from build123d import *

# Parameters (mm, degrees)
F0_W     = 203.2
F0_H     = 304.8
F0_W_2   = 125.476
F0_H_2   = 59.863002
F0_W_3   = 77.724
F0_H_3   = 58.935668
F1_DEPTH = 50.8


with BuildPart() as f1:
    # F0 (on Front) → F1 (new body)
    with BuildSketch(Plane.XZ):
        Rectangle(F0_W, F0_H)
        Polygon((-38.862, -109.735668), (-38.862, -50.8), (-62.738, -50.8), (-62.738, 54.436998), (-62.738, 114.3), (62.738, 114.3), (62.738, 54.436998), (62.738, -50.8), (38.862, -50.8), (38.862, -109.735668), align=None, mode=Mode.SUBTRACT)
        with Locations((0, 84.368499)):
            Rectangle(F0_W_2, F0_H_2)
        with Locations((0, -80.267834)):
            Rectangle(F0_W_3, F0_H_3)
    extrude(amount=F1_DEPTH)


solid = f1.part
Read the model definition and answer for the solid it produces. Units are mm, in the model's axes. A direction names the side the tool comes from. Give positions to 0.01 mm unless a question says otherwise; leave off trailing zeros. Write each loop counter-clockwise with the first axis right and the second up, starting at its lowest first coordinate (ties: lowest second). Pieces come first, ordered by that corner, then holes. Notation, with made-up numbers: M -12.75,71 L -8.75,71 A30 ccw -8.75,97 Z; hole C 89.25,15 d11. An arc over 180 degrees is marked long. One line per item, written item: value. Start each with the question number.
(1) Determine the mould class of faces 3 (the flat face through (66, -50.8, 2)), 4 (the flat face through (-1, -25, 152.4)), 5 (the flat face through (62.738, -25, 3)) for opening direction Z: pulls with the +Z half, pulls with the -Z half, needs draft (parallel to the pull), parting line crosses it, or undercut.
(2) Find section A-A (z = -1.5). Determine the outline of the cut face in (x, y), plus the area to 3 significant figures.
(3) A flat-ended cylindrical pin translates along its axis: pin 1 Ø10 at (x, z) = (-71, -84.5) entering from +Y. Find the tip coordinate at first contact, or state that the pin passes through.
(4) Find the intervals of material crossed by line 1 (Z direction, x = -23, y = -39.5); line 2 (X direction, y = -20.5, z = 31), in increasing order.
(5) Find section C-C (y = -16.5). Determine the outline of the cut face in (x, z), plus the area to 3 significant figures.
(6) A tool of negligible diameter and unlimited length cuts with its end or side. For faces 1 (the flat face through (66, 0, 2)), 2 (the flat face through (-1, -25, 54.437)), from which of +Z, -Z, +X, -X, +Y, -Y can it reach the whole face along a straight path? Write none if from no direction.
(7) Find section B-B (x = 13). Determine the outline of the cut face in (y, z), plus the area to 3 significant figures.
Results below:
1. face 3: needs draft
1. face 4: pulls with the +Z half
1. face 5: undercut
2. outline: M -101.6,-50.8 L -62.74,-50.8 L -62.74,0 L -101.6,0 Z; M 62.74,-50.8 L 101.6,-50.8 L 101.6,0 L 62.74,0 Z
2. area: 3,950 mm^2
3. pin 1: stops at y = 0
4. line 1: z = -152.4 to -50.8, 54.44 to 152.4
4. line 2: x = -101.6 to -62.74, 62.74 to 101.6
5. outline: M -101.6,-152.4 L 101.6,-152.4 L 101.6,152.4 L -101.6,152.4 Z; hole M -62.74,-50.8 L 62.74,-50.8 L 62.74,54.44 L -62.74,54.44 Z
5. area: 48,700 mm^2
6. face 1: +Z, -Z, +X, -X, +Y
6. face 2: +Y, -Y
7. outline: M -50.8,-152.4 L 0,-152.4 L 0,-50.8 L -50.8,-50.8 Z; M -50.8,54.44 L 0,54.44 L 0,152.4 L -50.8,152.4 Z
7. area: 10,100 mm^2
